Print and shaded views of the part. All mm, measured from the part's lowest x, y and z. A direction names the side the tool comes from. Coordinates: 2 decimals unless noted, no trailing zeros. Loops run counter-clockwise (first coordinate to the right, second up) from the corner with the lowest first, then second, coordinate; pieces in that order, holes last. Notation, with made-up numbers: (2, 29.5) -> (46, 29.5) arc R17 ccw to (46, 34.5) -> close; hole circle Ø10 at (52, -31.75). An arc over 180 degrees is marked (long way). One line per question, with ' | ' between items. Start each with the question number.
1) Two-plate mould, pull along Y, no slides. Class the marked faces 1, 2 and 3: released by +Y, released by -Y, zero draft, split by the parting line, or undercut.
2) 3-axis set-ups, long thin cutter, end or side, ignore diameter. For the marked faces 4 and 5: which of +Z, -Z, +X, -X, +Y, -Y reach the whole face in a straight line?
3) Cut at D-D (y = 19.75). List the corners of the cut face in (x, z) (1 decimal).
4) Probe L1, parallel to X at y = 5.5, z = 7.5; L2, parallel to X at y = 11.5, z = 3; L3, parallel to Z at x = 2, y = 9.5. List the from-to ranges inside material, lowest first. Write a range as from..to.
5) Drop flat-ended pins along their axis: pin 1 (6 mm diameter, centred on x = 7.5, y = 12, fed in from +Z); pin 2 (4 mm diameter, centred on x = 15.5, z = 4.5, fed in from -Y); pin 3 (4.5 mm diameter, centred on x = 3, y = 11, fed in from +Z); pin 4 (3 mm diameter, centred on x = 19, y = 11, fed in from +Z). Give the stop position or say it passes through.
6) Cut at A-A (x = 11). List the corners of the cut face in (y, z).
7) Cut at C-C (z = 2.5). List the corners of the cut face in (x, y).
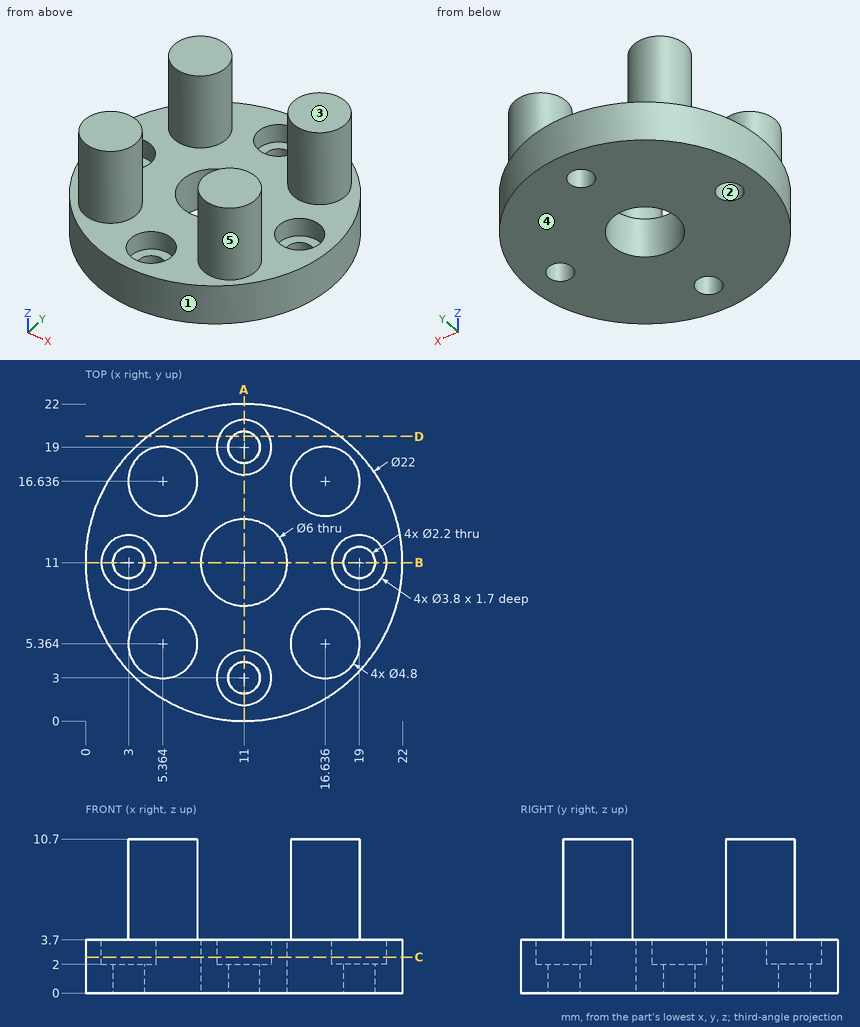
Reported:
1) face 1: split by the parting line | face 2: undercut | face 3: zero draft
2) face 4: -Z, +X, -X, +Y, -Y | face 5: +Z
3) outline: (4.3, 0) -> (10.2, 0) -> (10.2, 2) -> (9.3, 2) -> (9.3, 3.7) -> (4.3, 3.7) -> close; (11.8, 0) -> (17.7, 0) -> (17.7, 3.7) -> (12.7, 3.7) -> (12.7, 2) -> (11.8, 2) -> close
4) L1: x = 2.97..7.76, 14.24..19.03 | L2: x = 0.01..1.17, 4.83..8.04, 13.96..17.17, 20.83..21.99 | L3: z = 0..2
5) pin 1: stops at z = 10.7 | pin 2: stops at y = 0.33 | pin 3: stops at z = 3.7 | pin 4: stops at z = 2
6) outline: (0, 0) -> (1.9, 0) -> (1.9, 2) -> (1.1, 2) -> (1.1, 3.7) -> (0, 3.7) -> close; (4.1, 0) -> (8, 0) -> (8, 3.7) -> (4.9, 3.7) -> (4.9, 2) -> (4.1, 2) -> close; (14, 0) -> (17.9, 0) -> (17.9, 2) -> (17.1, 2) -> (17.1, 3.7) -> (14, 3.7) -> close; (20.1, 0) -> (22, 0) -> (22, 3.7) -> (20.9, 3.7) -> (20.9, 2) -> (20.1, 2) -> close
7) outline: circle Ø22 at (11, 11); hole circle Ø3.8 at (3, 11); hole circle Ø6 at (11, 11); hole circle Ø3.8 at (11, 3); hole circle Ø3.8 at (11, 19); hole circle Ø3.8 at (19, 11)
